The model under review builds one solid part; all positions refer to its coordinate system, in mm. A direction names the side the tool comes from. Coordinates: 2 decimals unless noted, no trailing zeros. Write each loop counter-clockwise with the first axis right and the second up, starting at its lowest first coordinate (ties: lowest second). Pieces come first, ordered by that corner, then holes. Notation, with made-up numbers: (42.5, 71.5) - (62.5, 71.5) arc R12 cw to (62.5, 91.5) - close; hole circle Ø1 at (24, 58). An arc over 180 degrees is marked (long way). Put each result on its own line as item: value. Start each with the question number.
Item 1: To check wall thickness, follow L1, parallel to X at y = 1, z = 0; L2, parallel to Z at x = 43, y = 33; L3, parallel to Y at x = -36, z = 21. State the ranges of each line that lie inside material, in increasing order. Write a range as [from, to].
Item 2: Machinability: for faces 1 (the face through (-0.77, 8.214, -20.666)), 2 (the face through (33, 2, 0)), 3 (the face through (-0.77, 1.97, 10.01)), which of the approach directions +Z, -Z, +X, -X, +Y, -Y give a long, thin tool a straight path to every point of the face, cutting with its end or side? Answer none if there is none.
Item 3: Consider section C-C on x = -19. Give the boundary of the cut face in (y, z), then the cut area to 3 significant figures.
Item 4: Consider section D-D on y = 124. Give the boundary of the cut face in (x, z).
Item 5: Consider section B-B on z = 14. Give the boundary of the cut face in (x, y), then the cut area to 3 significant figures.
Item 6: Mouldability with a two-part tool opening along X and no side actions: class faces 4 (the face through (37.442, 108.564, -34.86)), 5 (the face through (0, 124, 60)), 6 (the face through (42.968, 1.972, 37.53)) as pulls with the +X half, pulls with the -X half, needs draft (parallel to the pull), parting line crosses it, or undercut.
Item 7: Consider section A-A on z = 0. Give the boundary of the cut face in (x, y), then the cut area to 3 significant figures.
Item 8: For pin 1 (4.5 mm diameter, centred on x = -35, z = 0, fed in from +Y); pin 2 (2.5 mm diameter, centred on x = 44.74, z = 36.61, fed in from +Y); pin 3 (1.5 mm diameter, centred on x = 1.5, y = 73.5, fed in from +Z); pin 4 (5 mm diameter, centred on x = 12, z = -16, fed in from +Y), all flat-tipped, find the tip position at first contact; note any pin that passes through.
```python
from build123d import *

# Parameters (mm, degrees)
SKETCH1_R           = 2
BOSS_EXTRUDE1_DEPTH = 4
SKETCH2_W           = 110
SKETCH2_H           = 20
BOSS_EXTRUDE2_DEPTH = 135
SKETCH3_W           = 110
SKETCH3_H           = 8.547835338
BOSS_EXTRUDE3_DEPTH = 10
CHAMFER1_SIZE       = 10
SKETCH4_R           = 15
BOSS_EXTRUDE4_DEPTH = 85
CUT_EXTRUDE1_DEPTH  = 85


with BuildPart() as part:
    # Sketch1 → Boss-Extrude1 (new body)
    with BuildSketch(Plane(origin=(0, 0, 0), x_dir=(1, 0, 0), z_dir=(0, 1, 0))):
        with BuildLine():
            Line((35, -45), (55, -45))
            Line((55, -45), (55, 45))
            Line((55, 45), (-55, 45))
            Line((-55, 45), (-55, -45))
            Line((-55, -45), (-35, -45))
            ThreePointArc((-35, -45), (0, -10), (35, -45))
        make_face()
        with Locations(Location((-35, 0, 0), (0, 0, 270))):
            Circle(SKETCH1_R, mode=Mode.SUBTRACT)
        with Locations(Location((35, 0, 0), (0, 0, 270))):
            Circle(SKETCH1_R, mode=Mode.SUBTRACT)
        with Locations(Location((-44.742033595, -36.607118396, 0), (0, 0, 270))):
            Circle(SKETCH1_R, mode=Mode.SUBTRACT)
        with Locations(Location((44.742033595, -36.607118396, 0), (0, 0, 270))):
            Circle(SKETCH1_R, mode=Mode.SUBTRACT)
    extrude(amount=BOSS_EXTRUDE1_DEPTH)



with BuildPart() as body_2:
    # Sketch2 → Boss-Extrude2 (new body)
    with BuildSketch(Plane(origin=(0, 4, 0), x_dir=(1, 0, 0), z_dir=(0, 1, 0))):
        with Locations((0, 35)):
            Rectangle(SKETCH2_W, SKETCH2_H)
    extrude(amount=BOSS_EXTRUDE2_DEPTH)


with BuildPart() as part_1:
    add(part.part)

    add(body_2.part)  # Boss-Extrude3 merges body 2
    # Sketch3 → Boss-Extrude3 (add)
    with BuildSketch(Plane(origin=(0, 4, 0), x_dir=(1, 0, 0), z_dir=(0, 1, 0))):
        with Locations((0, 20.726082331)):
            Rectangle(SKETCH3_W, SKETCH3_H)
    extrude(amount=BOSS_EXTRUDE3_DEPTH)

    # Chamfer1
    # the kernel refuses this chamfer: 10 mm, written as the material it takes off along each edge
    with BuildSketch(Plane(origin=(-80.71682988, 14, -16.452164662), x_dir=(0, -0.9996219169112968, 0.027495876610586317), z_dir=(1, 0, 0))) as chamfer1_piece_1_section:
        Polygon((CHAMFER1_SIZE * 0.999621916911, CHAMFER1_SIZE * 0.0274958766106), (-CHAMFER1_SIZE * 0.0274958766106, CHAMFER1_SIZE * 0.999621916911), (0, 0), align=None)
    chamfer1_piece_1 = extrude(amount=161.433659759, mode=Mode.PRIVATE)
    chamfer1_piece_1 = split(chamfer1_piece_1, bisect_by=Plane(origin=(0, 4, -19.564208601), z_dir=(0, 1, 0)), keep=Keep.TOP, mode=Mode.PRIVATE)
    chamfer1_piece_1 = split(chamfer1_piece_1, bisect_by=Plane(origin=(0, 10.613146748, -25), z_dir=(0, 0, 1)), keep=Keep.TOP, mode=Mode.PRIVATE)
    add(chamfer1_piece_1, mode=Mode.SUBTRACT)

    # Sketch4 → Boss-Extrude4 (add)
    with BuildSketch(Plane.XY.offset(-25)):
        with Locations(Location((0, 124, 0), (0, 0, 90))):
            Circle(SKETCH4_R)
    extrude(amount=BOSS_EXTRUDE4_DEPTH)

    # Sketch5 → Cut-Extrude1 (cut)
    with BuildSketch(Plane.XY.offset(-25)):
        with BuildLine():
            Line((-55, 139), (-55, 75.773917669))
            ThreePointArc((-55, 75.773917669), (-37.156416489, 109.008847521), (-14.276626111, 139))
            Line((-14.276626111, 139), (-55, 139))
        make_face()
        with BuildLine():
            Line((55, 139), (55, 75.773917669))
            ThreePointArc((55, 75.773917669), (37.156416489, 109.008847521), (14.276626111, 139))
            Line((14.276626111, 139), (55, 139))
        make_face()
    extrude(amount=-CUT_EXTRUDE1_DEPTH, mode=Mode.SUBTRACT)


solid = part_1.part
```
Report:
1. L1: [-55, -37], [-33, 33], [37, 55]
1. L2: [-45, -25]
1. L3: [0, 4]
2. face 1: +Z, +X, -X
2. face 2: +Y, -Y
2. face 3: +Z, -Y
3. outline: (0, -45) - (133.57, -45) - (133.57, -25) - (12.55, -25) - (4, -16.45) - (4, 15.61) - (0, 15.61) - close
3. area: 2,870 mm²
4. outline: (-26.66, -45) - (26.66, -45) - (26.66, -25) - (15, -25) - (15, 60) - (-15, 60) - (-15, -25) - (-26.66, -25) - close
5. outline: (-55, 0) - (-16.25, 0) - (-16.25, 4) - (-55, 4) - close; circle Ø30 at (0, 124); (16.25, 0) - (55, 0) - (55, 4) - (16.25, 4) - close
5. area: 1,020 mm²
6. face 4: pulls with the +X half
6. face 5: needs draft
6. face 6: undercut
7. outline: (-55, 0) - (-37, 0) - (-37, 4) - (-55, 4) - close; (-33, 0) - (33, 0) - (33, 4) - (-33, 4) - close; circle Ø30 at (0, 124); (37, 0) - (55, 0) - (55, 4) - (37, 4) - close
7. area: 1,110 mm²
8. pin 1: y = 4
8. pin 2: through
8. pin 3: z = -25
8. pin 4: y = 135.61
